from build123d import *

# Parameters (mm, degrees)
F1_DEPTH = 51
F2_R     = 7.2426406871
F3_T     = 2.5


with BuildPart() as f1:
    # F0 (on Top) → F1 (new body)
    with BuildSketch(Plane.XY):
        with BuildLine():
            ThreePointArc((-66.1636230606, 59.9037967622), (-42.3757210374, 36.115894739), (-18.5878190141, 59.9037967622))
            Line((-18.5878190141, 59.9037967622), (-66.1636230606, 59.9037967622))
        make_face()
        with BuildLine():
            Line((-66.1636230606, 59.9037967622), (-18.5878190141, 59.9037967622))
            ThreePointArc((-18.5878190141, 59.9037967622), (-42.3757210374, 83.6916987855), (-66.1636230606, 59.9037967622))
        make_face()
        with BuildLine():
            Line((17.2835066915, 59.9037967622), (-18.5878190141, 59.9037967622))
            ThreePointArc((-18.5878190141, 59.9037967622), (-42.3757210374, 36.115894739), (-66.1636230606, 59.9037967622))
            Line((-66.1636230606, 59.9037967622), (-79.6502381563, 59.9037967622))
            Line((-79.6502381563, 59.9037967622), (-79.6502381563, -14.1544044018))
            Line((-79.6502381563, -14.1544044018), (17.2835066915, -14.1544044018))
            Line((17.2835066915, -14.1544044018), (17.2835066915, 59.9037967622))
        make_face()
    extrude(amount=F1_DEPTH)

    # F2
    f2_edges = [f1.edges().sort_by_distance(p)[0] for p in [
        (17.283507, 59.903797, 25.5),
        (-0.652156, 59.903797, 51),
        (17.283507, 22.874696, 51),
        (-42.375721, 83.691699, 51),
        (-72.906931, 59.903797, 51),
    ]]
    fillet(f2_edges, radius=F2_R)

    # F3
    f3_openings = [f1.faces().sort_by_distance(p)[0] for p in [
        (-31.290289, -14.154404, 25.445494),
        (-32.483683, 28.024527, 0),
    ]]
    offset(amount=F3_T, openings=f3_openings, kind=Kind.INTERSECTION)


solid = f1.part
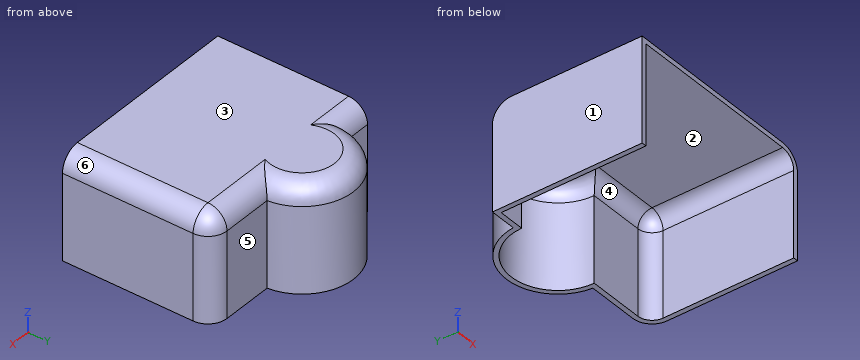
Geometry check sheet. Reference: the model listing, model coordinates, mm. Face numbers are marked on the shaded views. A direction names the side the tool comes from. Coordinates: 2 decimals unless noted, no trailing zeros. Order: outer loops, then holes, each group sorted by start corner. A loop starts at its lowest first (then second) coordinate and runs counter-clockwise, first axis right, second up. Notation, with made-up numbers: M -39.75,47.25 L -21.75,47.25 A25 ccw -21.75,71.25 Z; hole C 51.5,-40 d8. An arc over 180 degrees is marked long. Use CSV: the item, a comma, the result in double quotes.
Item 1: Thickness scan on line 1 along X through (y, z) = (6.5, 16); line 2 along Z through (x, y) = (0, 16); line 3 along X through (y, z) = (-0.5, 49). Record the ranges inside material, lowest first.
Returned:
line 1,"x = -82.15 to -79.65, 17.28 to 19.78"
line 2,"z = 51 to 53.5"
line 3,"x = -82.15 to -79.65, 15.04 to 18.25"
Item 2: Cross-section at C-C on y = 4. Record the cut outline in (x, z), then the cut area to 3 significant figures.
Returned:
outline,"M -82.15,0 L -79.65,0 L -79.65,51 L 10.04,51 A7.24 cw 17.28,43.76 L 17.28,0 L 19.78,0 L 19.78,43.76 A9.74 ccw 10.04,53.5 L -82.15,53.5 Z"
area,"501 mm2"
Item 3: Tool access check on the marked faces 4, 5 and 6. Record the directions out of +Z, -Z, +X, -X, +Y, -Y that give a thin tool (end or side, any length) a straight path to the whole face; none if there is none.
Returned:
face 4,"-Z, -Y"
face 5,"+Z, -Z, +X, +Y"
face 6,"+Z, +X, +Y, -Y"
Item 4: Gauge pin test, flat ends, axial feed: pin 1 Ø1.5 at (y, z) = (53, 46.5) entering from +X; pin 2 Ø10 at (y, z) = (75.5, 19.5) entering from -X; pin 3 Ø1.5 at (y, z) = (74.5, 43.5) entering from -X. Record the tip position at first contact, or that the pin passes through.
Returned:
pin 1,"stops at x = 19.57"
pin 2,"stops at x = -66.43"
pin 3,"stops at x = -64.72"
Item 5: Mould release check, pull along X, two halves, no side actions. Record for the marked faces 1, 2 and 3: pulls with the +X half, pulls with the -X half, needs draft (parallel to the pull), parting line crosses it, or undercut.
Returned:
face 1,"pulls with the -X half"
face 2,"undercut"
face 3,"needs draft"
Item 6: Cross-section at A-A on x = -71.5. Record the cut outline in (y, z), then the cut area to 3 significant figures.
Returned:
outline,"M -14.15,51 L 52.66,51 A7.24 cw 59.9,43.76 L 59.9,0 L 62.4,0 L 62.4,43.76 A9.74 ccw 52.66,53.5 L -14.15,53.5 Z"
area,"310 mm2"
